Work out the finished part from the listing and answer in its coordinate system (mm). A direction names the side the tool comes from. Round coordinates to 2 decimals unless told otherwise and drop trailing zeros. Loops run counter-clockwise (first coordinate to the right, second up) from the corner with the lowest first, then second, coordinate; pieces in that order, holes last. Notation, with made-up numbers: (32.5, -10.5) -> (63.5, -10.5) arc R14 cw to (63.5, 1.5) -> close; hole circle Ø7 at (48.5, -25.75). An arc over 180 degrees is marked (long way). Write item = value, one per line. Start each with the question number.
```python
from build123d import *

# Parameters (mm, degrees)
F0_W      = 56
F0_H      = 15
F1_DEPTH  = 37.5
F3_W      = 12
F3_H      = 63
F4_DEPTH  = 100
F6_DEPTH  = 43.501
F7_R      = 18
F8_DEPTH  = 25
F10_DEPTH = 43.501
F11_R     = 11
F12_DEPTH = 63.001
F2_W      = 32
F2_H      = 5
F13_DEPTH = 75.001
F14_R     = 6
F15_DEPTH = 15.001


with BuildPart() as f1:
    # F0 (on Front) → F1 (new body, symmetric)
    with BuildSketch(Plane.XZ):
        Rectangle(F0_W, F0_H)
    extrude(amount=F1_DEPTH, both=True)

    # F3 (on face) → F4 (join)
    with BuildSketch(Plane(origin=(-28, 0, 0), x_dir=(0, -1, 0), z_dir=(-1, 0, 0))):
        with Locations((0, 24)):
            Rectangle(F3_W, F3_H)
    extrude(amount=-F4_DEPTH)

    # F5 (on face) → F6 (cut, through all)
    with BuildSketch(Plane.XZ.offset(6)):
        Polygon((-28, 55.5), (-28, 7.5), (36.446944, 55.5), align=None)
    extrude(amount=-F6_DEPTH, mode=Mode.SUBTRACT)

    # F7 (on face) → F8 (join)
    with BuildSketch(Plane.XY.offset(55.5)):
        with Locations((72, 0)):
            Circle(F7_R)
    extrude(amount=-F8_DEPTH)

    # F9 (on face) → F10 (cut, through all)
    with BuildSketch(Plane.XZ.offset(6)):
        Polygon((55.029437, 30.5), (28, -7.5), (72, -7.5), (72, 30.5), align=None)
    extrude(amount=-F10_DEPTH, mode=Mode.SUBTRACT)

    # F11 (on face) → F12 (cut, through all)
    with BuildSketch(Plane.XY.offset(55.5)):
        with Locations((72, 0)):
            Circle(F11_R)
    extrude(amount=-F12_DEPTH, mode=Mode.SUBTRACT)

    # F2 (on face) → F13 (cut, through all)
    with BuildSketch(Plane.XZ.offset(37.5)):
        with Locations((0, -5)):
            Rectangle(F2_W, F2_H)
    extrude(amount=-F13_DEPTH, mode=Mode.SUBTRACT)

    # F14 (on face) → F15 (cut, through all)
    with BuildSketch(Plane.XY.offset(7.5)):
        with Locations((0, 22.5)):
            Circle(F14_R)
        with Locations((0, -22.5)):
            Circle(F14_R)
    extrude(amount=-F15_DEPTH, mode=Mode.SUBTRACT)


solid = f1.part
```
Item 1: Find the intervals of material crossed by line 1 along Y through (x, z) = (0, 1.75); line 2 along Y through (x, z) = (72, 35.75); line 3 along X through (y, z) = (-22, 0), in increasing order. Write a range as [from, to].
Item 2: A tool of negligible diameter and unlimited length cuts with its end or side. For faces 4 (the flat face through (0, -1, -2.5)), 5 (the flat face through (80, -8, 30.5)), 6 (the flat face through (28, 22, 0)), 7 (the flat face through (-7, -22, 7.5)), from which of +Z, -Z, +X, -X, +Y, -Y can it reach the whole face along a straight path? Write none if from no direction.
Item 3: Flat-ended cylindrical pins translate along their axes: pin 1 (10 mm diameter, centred on x = 6.5, z = 24, fed in from +Y); pin 2 (16 mm diameter, centred on x = 9, y = -18.5, fed in from +Z); pin 3 (10 mm diameter, centred on y = -23.5, z = 4.5, fed in from +X). Find the tip coordinate at first contact, or state that the pin passes through.
Item 4: Section B-B (x = 72) is taken. Determine the outline of the cut face in (y, z).
Item 5: Section A-A (y = 0) is taken. Determine the outline of the cut face in (x, z), then the cut area to 3 significant figures.
Item 6: Section D-D (z = 34) is taken. Determine the outline of the cut face in (x, y), then the cut area to 3 significant figures.
Item 7: The mould has two halves that part along Y. Classify faces 1 (the cylindrical face through (-1.301, -28.357, 2.57)), 2 (the cylindrical face through (89.986, -0.706, 43.175)), 3 (the flat face through (-16, -1, -5)): pulls with the +Y half, pulls with the -Y half, needs draft (parallel to the pull), parting line crosses it, or undercut.
Item 8: Section C-C (x = 0) is taken. Determine the outline of the cut face in (y, z).
Worked answers:
q1.line_1 = [-37.5, -28.5], [-16.5, 16.5], [28.5, 37.5]
q1.line_2 = [-18, -11], [11, 18]
q1.line_3 = [-28, -5.98], [5.98, 28]
q2.face_4 = -Z, +Y, -Y
q2.face_5 = -Z, +X, +Y, -Y
q2.face_6 = +Z, -Z, +X, +Y
q2.face_7 = +Z, +X, -X, -Y
q3.pin_1 = 6
q3.pin_2 = 7.5
q3.pin_3 = 28
q4.outline = (-18, 30.5) -> (-11, 30.5) -> (-11, 55.5) -> (-18, 55.5) -> close; (11, 30.5) -> (18, 30.5) -> (18, 55.5) -> (11, 55.5) -> close
q5.outline = (-28, -7.5) -> (-16, -7.5) -> (-16, -2.5) -> (16, -2.5) -> (16, -7.5) -> (28, -7.5) -> (55.03, 30.5) -> (61, 30.5) -> (61, 55.5) -> (36.45, 55.5) -> (-28, 7.5) -> close; (83, 30.5) -> (90, 30.5) -> (90, 55.5) -> (83, 55.5) -> close
q5.area = 3,330 mm2
q6.outline = (7.58, -6) -> (55.03, -6) arc R18 ccw (long way) to (55.03, 6) -> (7.58, 6) -> close; hole circle Ø22 at (72, 0)
q6.area = 1,200 mm2
q7.face_1 = undercut
q7.face_2 = parting line crosses it
q7.face_3 = needs draft
q8.outline = (-37.5, -2.5) -> (-28.5, -2.5) -> (-28.5, 7.5) -> (-37.5, 7.5) -> close; (-16.5, -2.5) -> (16.5, -2.5) -> (16.5, 7.5) -> (6, 7.5) -> (6, 28.35) -> (-6, 28.35) -> (-6, 7.5) -> (-16.5, 7.5) -> close; (28.5, -2.5) -> (37.5, -2.5) -> (37.5, 7.5) -> (28.5, 7.5) -> close
